Design review of the part built by this model. Coordinates are the model's own, in mm. Coordinates: 2 decimals unless noted, no trailing zeros. Order: outer loops, then holes, each group sorted by start corner. A loop starts at its lowest first (then second) coordinate and runs counter-clockwise, first axis right, second up. Notation, with made-up numbers: (87, -28.5) -> (118, -28.5) arc R26 ccw to (118, 5.5) -> close; hole circle Ø6 at (54.5, -27). An arc over 180 degrees is marked (long way). Use a Markdown table: item, result. Add a question column.
Q1. Wall thickness on probe 1 along Y at (x, z) = (-10.5, 1.95); probe 2 along Y at (x, z) = (54.5, 0.95); probe 3 along Y at (x, z) = (-18.5, 1.6): over which ranges is each line inside the solid? List them lowest first.
Q2. Add section B-B (y = 90.5). State the section outline as (x, z) points, then the cut area to 3 significant figures.
Q3. Add section D-D (z = 0.85). Count the separate pieces of the cut face and the enclosed holes in it, then the cut area to 3 significant figures.
Q4. Add section C-C (y = 2). State the section outline as (x, z) points.
Q5. Add section A-A (x = 49). State the section outline as (y, z) points.
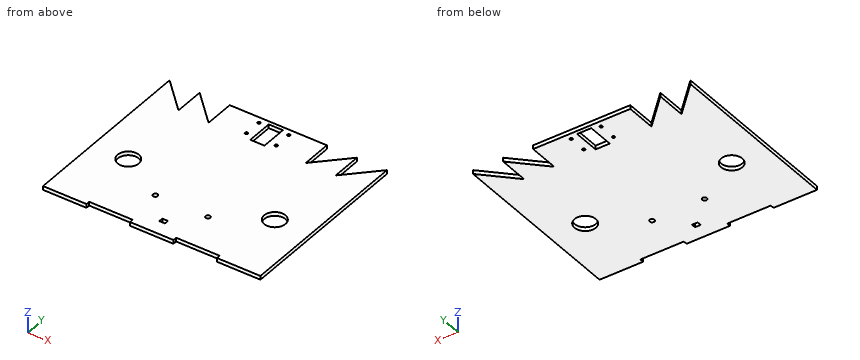
from build123d import *

# Parameters (mm, degrees)
SKETCH1_R           = 1.65
SKETCH1_R_2         = 7.5
SKETCH1_R_3         = 1
SKETCH1_W           = 4
SKETCH1_H           = 3
SKETCH1_W_2         = 10
SKETCH1_H_2         = 18.5
BOSS_EXTRUDE3_DEPTH = 2.7


with BuildPart() as part:
    # Sketch1 → Boss-Extrude3 (new body)
    with BuildSketch(Plane.XY):
        Polygon((-46.02, -28), (-46.02, -25.3), (-15.34, -25.3), (-15.34, -28), (15.34, -28), (15.34, -25.3), (46.02, -25.3), (46.02, -28), (76.7, -28), (76.7, 99), (55.486796564, 77.786796564), (55.486796564, 99), (34.273593129, 77.786796564), (34.273593129, 99), (-34.273593129, 99), (-34.273593129, 77.786796564), (-55.486796564, 99), (-55.486796564, 77.786796564), (-76.7, 99), (-76.7, -28), align=None)
        with Locations((-18.5, 2)):
            Circle(SKETCH1_R, mode=Mode.SUBTRACT)
        with Locations((18.567940233, 2)):
            Circle(SKETCH1_R, mode=Mode.SUBTRACT)
        with Locations((-51.7, 22)):
            Circle(SKETCH1_R_2, mode=Mode.SUBTRACT)
        with Locations((51.7, 22)):
            Circle(SKETCH1_R_2, mode=Mode.SUBTRACT)
        with Locations((10.5, 94.5)):
            Circle(SKETCH1_R_3, mode=Mode.SUBTRACT)
        with Locations((-10.5, 82)):
            Circle(SKETCH1_R_3, mode=Mode.SUBTRACT)
        with Locations((-10.5, 94.5)):
            Circle(SKETCH1_R_3, mode=Mode.SUBTRACT)
        with Locations((10.5, 82)):
            Circle(SKETCH1_R_3, mode=Mode.SUBTRACT)
        with Locations((0, -16)):
            Rectangle(SKETCH1_W, SKETCH1_H, mode=Mode.SUBTRACT)
        with Locations((0, 87.25)):
            Rectangle(SKETCH1_W_2, SKETCH1_H_2, mode=Mode.SUBTRACT)
    extrude(amount=BOSS_EXTRUDE3_DEPTH)


solid = part.part
Established:
| question | item | result |
|---|---|---|
| 1 | probe 1 | -28 to 81, 83 to 93.5, 95.5 to 99 |
| 1 | probe 2 | -28 to 15.04, 28.96 to 98.01 |
| 1 | probe 3 | -25.3 to 0.35, 3.65 to 99 |
| 2 | outline | (-76.7, 0) -> (-68.2, 0) -> (-68.2, 2.7) -> (-76.7, 2.7) -> close; (-55.49, 0) -> (-46.99, 0) -> (-46.99, 2.7) -> (-55.49, 2.7) -> close; (-34.27, 0) -> (-5, 0) -> (-5, 2.7) -> (-34.27, 2.7) -> close; (5, 0) -> (34.27, 0) -> (34.27, 2.7) -> (5, 2.7) -> close; (46.99, 0) -> (55.49, 0) -> (55.49, 2.7) -> (46.99, 2.7) -> close; (68.2, 0) -> (76.7, 0) -> (76.7, 2.7) -> (68.2, 2.7) -> close |
| 2 | area | 250 mm^2 |
| 3 | separate pieces | 1 |
| 3 | enclosed holes | 10 |
| 3 | area | 17,800 mm^2 |
| 4 | outline | (-76.7, 0) -> (-20.15, 0) -> (-20.15, 2.7) -> (-76.7, 2.7) -> close; (-16.85, 0) -> (16.92, 0) -> (16.92, 2.7) -> (-16.85, 2.7) -> close; (20.22, 0) -> (76.7, 0) -> (76.7, 2.7) -> (20.22, 2.7) -> close |
| 5 | outline | (-28, 0) -> (15, 0) -> (15, 2.7) -> (-28, 2.7) -> close; (29, 0) -> (92.51, 0) -> (92.51, 2.7) -> (29, 2.7) -> close |
